Input: part model. Units: mm. Frame: model coordinates. Face numbers are marked on the shaded views. A direction names the side the tool comes from. Round coordinates to 2 decimals unless told otherwise and drop trailing zeros. Loops run counter-clockwise (first coordinate to the right, second up) from the corner with the lowest first, then second, coordinate; pieces in that order, holes last. Notation, with made-up numbers: M 78,-16 L 107,-16 A26 ccw 107,-2 Z; hole C 80,78 d2. An arc over 180 degrees is marked long. Return JSON: item names as keys, results as strings. Group by question number.
1) Section D-D (z = 40.5). Output: boundary loops of the cut face in (x, y).
2) Section A-A (x = -8.25). Output: boundary loops of the cut face in (y, z), plus the area to 3 significant figures.
3) Section C-C (z = 18). Output: boundary loops of the cut face in (x, y), plus the area to 3 significant figures.
4) Access query for the marked faces 1, 2 and 3. Directions: +Z, -Z, +X, -X, +Y, -Y. A direction counts if a zero-diameter tool reaches every point of the face in a straight line with its end or side. Return the directions, or none.
5) Contact query for flat-ended pins moving along their axis: P1, Ø6, axis at y = -1.5, z = 34.5, coming from the -X side; P2, Ø0.5, axis at x = 0, y = 0.5, coming from the +Z side; P3, Ø1, axis at x = -1, y = -10, coming from the +Z side; P4, Ø3, axis at y = -20, z = 28.5, coming from the +X side. Output: stop coordinate, or through.
6) Material intervals for line 1 (Y direction, x = 0, z = 40.25); line 2 (Z direction, x = -4.5, y = -7.5); line 3 (Z direction, x = -7, y = 6), sorted ascending. Write a range as from..to.
7) Section B-B (y = -4). Output: boundary loops of the cut face in (x, z).
8) Mould query, pull axis Z, two halves, no side actions, for the marked faces 4, 5 and 6. Classes: +Z half, -Z half, draft (parallel to the pull), parting line (faces both ways), or undercut.
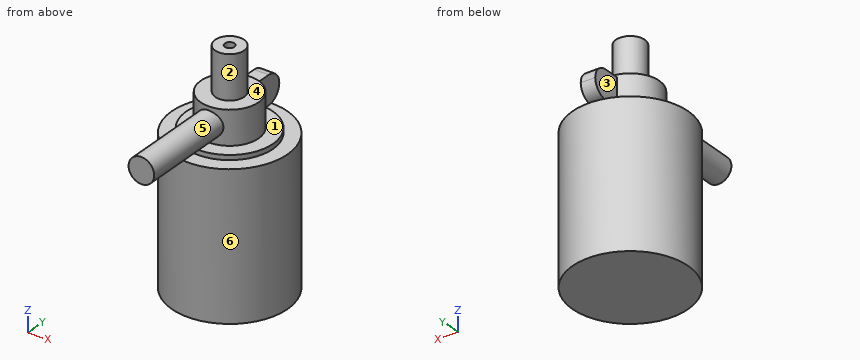
from build123d import *

# Parameters (mm, degrees)
F0_R         = 12
F1_DEPTH     = 30
F2_R         = 9
F3_DEPTH     = 1
F4_R         = 6
F5_DEPTH     = 7
F6_R         = 3
F7_DEPTH     = 9
F8_R         = 1
F9_DEPTH     = 25
F10_R        = 2.6468455099
F11_DEPTH    = 25
F12_W        = 3
F12_H        = 5.9210534014
F13_DEPTH    = 12
F14_T1_DEPTH = 18


# Not quite as in the source:
# - a fillet or chamfer that OpenCascade refuses, or shapes differently, is made with other operations: its cross-section is extruded or revolved along the edge and cut away or added


with BuildPart() as f1:
    # F0 (on Top) → F1 (new body)
    with BuildSketch(Plane.XY):
        Circle(F0_R)
    extrude(amount=F1_DEPTH)

    # F2 (on face) → F3 (join)
    with BuildSketch(Plane.XY.offset(30)):
        Circle(F2_R)
    extrude(amount=F3_DEPTH)

    # F4 (on face) → F5 (join)
    with BuildSketch(Plane.XY.offset(31)):
        Circle(F4_R)
    extrude(amount=F5_DEPTH)

    # F6 (on face) → F7 (join)
    with BuildSketch(Plane.XY.offset(38)):
        Circle(F6_R)
    extrude(amount=F7_DEPTH)

    # F8 (on face) → F9 (cut)
    with BuildSketch(Plane.XY.offset(47)):
        Circle(F8_R)
    extrude(amount=-F9_DEPTH, mode=Mode.SUBTRACT)

    # F10 (on Front) → F11 (join)
    with BuildSketch(Plane.XZ):
        with Locations((0, 34.5747359097)):
            Circle(F10_R)
    extrude(amount=F11_DEPTH)

    # F12 (on Front) → F13 (join)
    with BuildSketch(Plane.XZ):
        with Locations((0, 34.5066897571)):
            Rectangle(F12_W, F12_H)
    extrude(amount=-F13_DEPTH)

    # F14: fillet of radius 3 on 2 edges, made by hand

    # F14_s2 → F14_t1 (cut)
    with BuildSketch(Plane.YZ.offset(-9)):
        with BuildLine():
            ThreePointArc((9, 37.4672164578), (11.1213203436, 36.5885368014), (12, 34.4672164578))
            Line((12, 34.4672164578), (12, 37.4672164578))
            Line((12, 37.4672164578), (9, 37.4672164578))
        make_face()
        with BuildLine():
            ThreePointArc((9, 31.5461630564), (11.1213203436, 32.4248427128), (12, 34.5461630564))
            Line((12, 34.5461630564), (12, 31.5461630564))
            Line((12, 31.5461630564), (9, 31.5461630564))
        make_face()
    extrude(amount=F14_T1_DEPTH, mode=Mode.SUBTRACT)


solid = f1.part
Returned:
{
 "1": {"outline": "C 0,0 d6; hole C 0,0 d2"},
 "2": {"outline": "M -8.71,0 L 8.71,0 L 8.71,30 L 3.6,30 L 3.6,31 L -3.6,31 L -3.6,30 L -8.71,30 Z", "area": "530 mm^2"},
 "3": {"outline": "C 0,0 d24", "area": "452 mm^2"},
 "4": {"face 1": "none", "face 2": "+Z", "face 3": "+Z, -X, +Y"},
 "5": {"P1": "stops at x = -6", "P2": "stops at z = 37.47", "P3": "stops at z = 37.17", "P4": "passes through"},
 "6": {"line 1": "y = -3..-1, 1..3", "line 2": "z = 0..31", "line 3": "z = 0..30"},
 "7": {"outline": "M -11.31,0 L 11.31,0 L 11.31,30 L 8.06,30 L 8.06,31 L 4.47,31 L 4.47,38 L -4.47,38 L -4.47,31 L -8.06,31 L -8.06,30 L -11.31,30 Z"},
 "8": {"face 4": "+Z half", "face 5": "undercut", "face 6": "draft"}
}
